from build123d import *

# Parameters (mm, degrees)
RESSALTO_EXTRUS_O1_DEPTH = 2
ESBO_O2_W                = 4
ESBO_O2_H                = 2.8
RESSALTO_EXTRUS_O2_DEPTH = 7


with BuildPart() as part:
    # Esboço1 → Ressalto-extrusão1 (new body)
    with BuildSketch(Plane.XY):
        Polygon((-10, 0), (-10, 7), (13, 7), (13, -5), (5, -5), (0, 0), align=None)
    extrude(amount=RESSALTO_EXTRUS_O1_DEPTH)

    # Esboço2 → Ressalto-extrusão2 (add)
    with BuildSketch(Plane.XY.offset(2)):
        with BuildLine():
            Line((13, 7), (-4, 7))
            Line((-4, 7), (-4, 5))
            Line((-4, 5), (7.7, 5))
            ThreePointArc((7.7, 5), (11.546036921, -1.223018461), (4.26, -1.88))
            Line((4.26, -1.88), (1.8, 1.4))
            ThreePointArc((1.8, 1.4), (1.094427191, 1.988854382), (0.2, 2.2))
            Line((0.2, 2.2), (-10, 2.2))
            Line((-10, 2.2), (-10, 0))
            Line((-10, 0), (0, 0))
            Line((0, 0), (5, -5))
            Line((5, -5), (13, -5))
            Line((13, -5), (13, 7))
        make_face()
        with Locations((-8, 5.6)):
            Rectangle(ESBO_O2_W, ESBO_O2_H)
        with BuildLine():
            Line((7.7, 3.2), (6.7, 3.2))
            ThreePointArc((6.7, 3.2), (4.911145618, 2.094427191), (5.1, 0))
            Line((5.1, 0), (5.7, -0.8))
            ThreePointArc((5.7, -0.8), (9.936067977, -0.418033989), (7.7, 3.2))
        make_face()
    extrude(amount=RESSALTO_EXTRUS_O2_DEPTH)


solid = part.part
Here's how the part is built. I have some questions about the finished solid (model axes, mm). A direction names the side the tool comes from. Give positions to 0.01 mm unless a question says otherwise; leave off trailing zeros. Order: outer loops, then holes, each group sorted by start corner. A loop starts at its lowest first (then second) coordinate and runs counter-clockwise, first axis right, second up. Notation, with made-up numbers: (-8.5, 80.25) -> (14.5, 80.25) arc R24 cw to (14.5, 107.25) -> close; hole circle Ø7 at (37.25, -30). An arc over 180 degrees is marked (long way). One line per item, written item: value. Start each with the question number.
1. Will these pins go through, and if not, where does the flat tip stop? pin 1 Ø4.5 at (x, z) = (-7.5, 6.5) entering from -Y; pin 2 Ø1.5 at (x, y) = (2, 3.5) entering from +Z; pin 3 Ø1 at (x, y) = (-2.5, 2.5) entering from -Z; pin 4 Ø5 at (x, z) = (-0.5, 6.5) entering from -Y.
2. I need wall thicknesses on probe 1 along Y at (x, z) = (7.7, 6.5); probe 2 along X at (y, z) = (0.75, 5.5); probe 3 along Y at (x, z) = (-9, 3.5). Which ranges of each line are inside material? Lowest first, please. Write a range as from..to.
3. For faces 5 (the face through (-5, 2.2, 5)), 6 (the face through (-5, 0, 4)), 7 (the face through (-6, 6, 5)), 8 (the face through (5.4, -0.4, 5.5)), which set-ups out of +Z, -Z, +X, -X, +Y, -Y let a thin tool reach every point of the face, with its end or its side?
4. Imagine slicing it at D-D, the plane z = 1. List the corners of the cut face in (x, y) for me, plus the area to 4 significant figures.
5. Imagine slicing it at C-C, the plane x = 3.75. List the corners of the cut face in (y, z) for me.
6. Imagine slicing it at B-B, the plane z = 3. List the corners of the cut face in (x, y) for me, plus the area to 3 significant figures.
7. Imagine slicing it at A-A, the plane y = 5.25. List the corners of the cut face in (x, z) for me.
8. We'd pull the mould along X, two halves only. Please class faces 1 (the face through (2, -2, 4)), 2 (the face through (13, 1, 4)), 3 (the face through (1.11, 1.98, 5.45)), 4 (the face through (-4, 6, 5)): released by +X, released by -X, zero draft, split by the parting line, or undercut.
Values follow:
1. pin 1: stops at y = 0
1. pin 2: stops at z = 2
1. pin 3: stops at z = 0
1. pin 4: stops at y = -2
2. probe 1: y = -5..-3.6, -1.8..3.2, 5..7
2. probe 2: x = -10..2.29, 4.75..10.2, 12..13
2. probe 3: y = 0..2.2, 4.2..7
3. face 5: +Z, -X
3. face 6: +Z, -Z, -X, -Y
3. face 7: +Z, +Y
3. face 8: +Z
4. outline: (-10, 0) -> (0, 0) -> (5, -5) -> (13, -5) -> (13, 7) -> (-10, 7) -> close
4. area: 213.5 mm2
5. outline: (-3.75, 0) -> (7, 0) -> (7, 9) -> (5, 9) -> (5, 2) -> (-1.2, 2) -> (-1.2, 9) -> (-3.75, 9) -> close
6. outline: (-10, 0) -> (0, 0) -> (5, -5) -> (13, -5) -> (13, 7) -> (-4, 7) -> (-4, 5) -> (7.7, 5) arc R4.3 cw (long way) to (4.26, -1.88) -> (1.8, 1.4) arc R2 ccw to (0.2, 2.2) -> (-10, 2.2) -> close; (-10, 4.2) -> (-6, 4.2) -> (-6, 7) -> (-10, 7) -> close; (5.1, 0) -> (5.7, -0.8) arc R2.5 ccw (long way) to (7.7, 3.2) -> (6.7, 3.2) arc R2 ccw to start
6. area: 131 mm2
7. outline: (-10, 0) -> (13, 0) -> (13, 9) -> (-4, 9) -> (-4, 2) -> (-6, 2) -> (-6, 9) -> (-10, 9) -> close
8. face 1: released by -X
8. face 2: released by +X
8. face 3: undercut
8. face 4: undercut
